Can you work these out from the model? Positions are in its coordinate system, mm. A direction names the side the tool comes from. Coordinates: 2 decimals unless noted, no trailing zeros. Order: outer loops, then holes, each group sorted by start corner. A loop starts at its lowest first (then second) coordinate and runs counter-clockwise, first axis right, second up.
```python
from build123d import *
from OCP.BRepFilletAPI import BRepFilletAPI_MakeChamfer

# Parameters (mm, degrees)
SKETCH1_W                       = 50
SKETCH1_H                       = 15
BOSS_EXTRUDE1_DEPTH             = 5
BOSS_EXTRUDE2_DEPTH             = 15
FILLET1_R                       = 2
SKETCH3_W                       = 80
SKETCH3_H                       = 15
BOSS_EXTRUDE3_DEPTH             = 3
CHAMFER1_SIZE                   = 2
CHAMFER1_SIZE2                  = 1.633074145
F_3_0MM_DOWEL_HOLE1_D           = 3
F_3_0MM_DOWEL_HOLE1_DEPTH       = 20
F_3_0MM_DOWEL_HOLE1_CSINK_D     = 3.05
F_3_0MM_DOWEL_HOLE1_CSINK_ANGLE = 90
F_3_0MM_DOWEL_HOLE1_TIP         = 0.901290929
F_2_5MM_DOWEL_HOLE1_D           = 2.5
F_2_5MM_DOWEL_HOLE1_DEPTH       = 20
F_2_5MM_DOWEL_HOLE1_CSINK_D     = 2.55
F_2_5MM_DOWEL_HOLE1_CSINK_ANGLE = 90
F_2_5MM_DOWEL_HOLE1_TIP         = 0.751075774


with BuildPart() as part:
    # Sketch1 → Boss-Extrude1 (new body)
    with BuildSketch(Plane(origin=(0, 0, 0), x_dir=(1, 0, 0), z_dir=(0, 1, 0))):
        Rectangle(SKETCH1_W, SKETCH1_H)
    extrude(amount=BOSS_EXTRUDE1_DEPTH)

    # Sketch2 → Boss-Extrude2 (add)
    with BuildSketch(Plane.XY.offset(7.5)):
        Polygon((25, 0), (40, -56), (35, -56), (20, 0), align=None)
        Polygon((-25, 0), (-40, -56), (-35, -56), (-20, 0), align=None)
    extrude(amount=-BOSS_EXTRUDE2_DEPTH)

    # Fillet1
    fillet1_edges = [part.edges().sort_by_distance(p)[0] for p in [
        (20, 0, 0),
        (-20, 0, 0),
    ]]
    fillet(fillet1_edges, radius=FILLET1_R)

    # Sketch3 → Boss-Extrude3 (add)
    with BuildSketch(Plane.XZ.offset(56)):
        Rectangle(SKETCH3_W, SKETCH3_H)
    extrude(amount=BOSS_EXTRUDE3_DEPTH)

    # Chamfer1: one chamfer whose edges measure the first distance from different faces: ONE call of the kernel's chamfer builder (chamfer() names one face for all edges)
    chamfer1_edges_1 = [part.edges().sort_by_distance(p)[0] for p in [
        (35, -56, 0),
    ]]
    chamfer1_side_1 = [part.faces().sort_by_distance(p)[0] for p in [
        (0, -56, 0),
    ]]
    chamfer1_edges_2 = [part.edges().sort_by_distance(p)[0] for p in [
        (-35, -56, 0),
    ]]
    chamfer1_side_2 = [part.faces().sort_by_distance(p)[0] for p in [
        (-27.698552834, -28.741263915, 0),
    ]]
    chamfer1 = BRepFilletAPI_MakeChamfer(part.part.solid().wrapped)
    for e in chamfer1_edges_1:
        chamfer1.Add(CHAMFER1_SIZE, CHAMFER1_SIZE2, e.wrapped, chamfer1_side_1[0].wrapped)  # the first distance lies on this face
    for e in chamfer1_edges_2:
        chamfer1.Add(CHAMFER1_SIZE, CHAMFER1_SIZE2, e.wrapped, chamfer1_side_2[0].wrapped)  # the first distance lies on this face
    add(Compound.cast(chamfer1.Shape()), mode=Mode.REPLACE)

    # Ø3.0mm Dowel Hole1
    with Locations(Plane(origin=(0, -56, 0), x_dir=(1, 0, 0), z_dir=(0, 1, 0))):
        with Locations((-25, 0), (25, 0)):
            CounterSinkHole(F_3_0MM_DOWEL_HOLE1_D / 2, F_3_0MM_DOWEL_HOLE1_CSINK_D / 2, depth=F_3_0MM_DOWEL_HOLE1_DEPTH, counter_sink_angle=F_3_0MM_DOWEL_HOLE1_CSINK_ANGLE)
            with Locations((0, 0, -(F_3_0MM_DOWEL_HOLE1_DEPTH + F_3_0MM_DOWEL_HOLE1_TIP / 2))):  # 118° drill point
                Cone(0, F_3_0MM_DOWEL_HOLE1_D / 2, F_3_0MM_DOWEL_HOLE1_TIP, mode=Mode.SUBTRACT)

    # Ø2.5mm Dowel Hole1
    with Locations(Plane(origin=(0, 5, 0), x_dir=(1, 0, 0), z_dir=(0, 1, 0))):
        with Locations((-12.05, 0), (12.05, 0)):
            CounterSinkHole(F_2_5MM_DOWEL_HOLE1_D / 2, F_2_5MM_DOWEL_HOLE1_CSINK_D / 2, depth=F_2_5MM_DOWEL_HOLE1_DEPTH, counter_sink_angle=F_2_5MM_DOWEL_HOLE1_CSINK_ANGLE)
            with Locations((0, 0, -(F_2_5MM_DOWEL_HOLE1_DEPTH + F_2_5MM_DOWEL_HOLE1_TIP / 2))):  # 118° drill point
                Cone(0, F_2_5MM_DOWEL_HOLE1_D / 2, F_2_5MM_DOWEL_HOLE1_TIP, mode=Mode.SUBTRACT)


solid = part.part
```
1. I'm going to push flat-ended pins straight in: pin 1 (2 mm diameter, centred on y = -17, z = 2, fed in from -X); pin 2 (1.5 mm diameter, centred on y = 1.5, z = 3, fed in from -X); pin 3 (8 mm diameter, centred on y = -33, z = -5, fed in from -X); pin 4 (3.5 mm diameter, centred on x = -25, z = 0, fed in from -Y). Where does each tip first touch, or does it pass through?
Completed:
pin 1: stops at x = -29.82
pin 2: stops at x = -25
pin 3: stops at x = -34.91
pin 4: stops at y = -59
2. Imagine slicing it at C-C on y = -19. Please give me the cut outline in (x, z).
Completed:
outline: (-30.09, -7.5) - (-25.09, -7.5) - (-25.09, 7.5) - (-30.09, 7.5) - close; (25.09, -7.5) - (30.09, -7.5) - (30.09, 7.5) - (25.09, 7.5) - close
3. Thinking about a two-plate mould opening in X: for faces 4 (the flat face through (-27, -24, -7.5)), 5 (the flat face through (-33.917, -55.048, 0.105)), 6 (the flat face through (-32.395, -27.608, 0.105)), which applies, pulls with the +X half, pulls with the -X half, needs draft (parallel to the pull), parting line crosses it, or undercut?
Completed:
face 4: needs draft
face 5: undercut
face 6: pulls with the -X half
4. Please list where these lines run through material, in increasing order: probe 1 along Z at (x, y) = (25, -58); probe 2 along Y at (x, z) = (-18.5, 0); probe 3 along X at (y, z) = (-46, 3.75).
Completed:
probe 1: z = -7.5 to -1.5, 1.5 to 7.5
probe 2: y = -59 to -56, 0 to 5
probe 3: x = -37.32 to -32.32, 32.32 to 37.32
5. Imagine slicing it at A-A on x = -12.05. Please give me the cut outline in (y, z) (3 decimals), then the cut area to 3 significant figures.
Completed:
outline: (-59, -7.5) - (-56, -7.5) - (-56, 7.5) - (-59, 7.5) - close; (0, -7.5) - (5, -7.5) - (5, -1.275) - (4.975, -1.25) - (0, -1.25) - close; (0, 1.25) - (4.975, 1.25) - (5, 1.275) - (5, 7.5) - (0, 7.5) - close
area: 107 mm2
6. On a 3-axis mill with a long thin cutter (end or side, diameter ignored), from which of +Z, -Z, +X, -X, +Y, -Y can I reach the whole of each face in a straight line? I mean faces 1 (the flat face through (-27.538, -28.143, 0.105)), 2 (the cylindrical face through (-23.5, -57.53, -0.07)), 3 (the cylindrical face through (10.895, 2.453, 0.479)). Say none if no direction works.
Completed:
face 1: +Z, -Z
face 2: -Y
face 3: +Y
7. Imagine slicing it at B-B on z = -2.75. Please give me the cut outline in (x, y), then the cut area to 3 significant figures.
Completed:
outline: (-40, -59) - (40, -59) - (40, -56) - (25, 0) - (25, 5) - (-25, 5) - (-25, 0) - (-40, -56) - close; hole (-34.48, -54.07) - (-33.37, -56) - (33, -56) - (34.58, -54.42) - (20.4, -1.48) arc R2 ccw to (18.47, 0) - (-18.47, 0) arc R2 ccw to (-20.4, -1.48) - close
area: 1,050 mm2
8. Imagine slicing it at D-D on x = 28. Please give me the cut outline in (y, z).
Completed:
outline: (-59, -7.5) - (-56, -7.5) - (-56, 7.5) - (-59, 7.5) - close; (-29.87, -7.5) - (-11.2, -7.5) - (-11.2, 7.5) - (-29.87, 7.5) - close
